Source: CAD feature listing. Evaluate the final solid. Frame: model axes, mm. Coordinates: 2 decimals unless noted, no trailing zeros. Loops run counter-clockwise (first coordinate to the right, second up) from the corner with the lowest first, then second, coordinate; pieces in that order, holes last. Notation, with made-up numbers: (-13.5, 16.25) -> (40.5, 16.25) arc R31 ccw to (40.5, 51.25) -> close; hole circle Ø11 at (-24, 13.5). An arc over 180 degrees is marked (long way). Answer as CSV lines item,"result".
from build123d import *

# Parameters (mm, degrees)
F1_DEPTH = 12
F3_DEPTH = 25
F5_D     = 5


with BuildPart() as f1:
    # F0 (on Front) → F1 (new body)
    with BuildSketch(Plane.XZ):
        with BuildLine():
            ThreePointArc((-6.1837801054, 11.6114190374), (-6.2418651063, 12.0437074429), (-6.411999761, 12.4453308138))
            ThreePointArc((-6.411999761, 12.4453308138), (-7.8214415512, 11.6114190374), (-9.1238598826, 10.6186242444))
            ThreePointArc((-9.1238598826, 10.6186242444), (-7.2975070499, 10.0598302873), (-6.1837801054, 11.6114190374))
        make_face()
        with BuildLine():
            ThreePointArc((-9.1238598826, 10.6186242444), (-5.8423437781, -12.7226970088), (14, 0))
            ThreePointArc((14, 0), (7.2880725623, 11.9534094854), (-6.411999761, 12.4453308138))
            ThreePointArc((-6.411999761, 12.4453308138), (-6.2418651063, 12.0437074429), (-6.1837801054, 11.6114190374))
            ThreePointArc((-6.1837801054, 11.6114190374), (-7.2975070499, 10.0598302873), (-9.1238598826, 10.6186242444))
        make_face()
    extrude(amount=F1_DEPTH)

    # F2 (on face) → F3 (cut)
    with BuildSketch(Plane.XZ.offset(12)):
        with BuildLine():
            ThreePointArc((-10.4471785382, 9.3196813567), (-8.7916106337, 8.9938043215), (-7.8551114747, 10.3973962329))
            ThreePointArc((-7.8551114747, 10.3973962329), (-7.9419845398, 10.903914247), (-8.1926740651, 11.3525367942))
            ThreePointArc((-8.1926740651, 11.3525367942), (-9.3751880821, 10.3973962329), (-10.4471785382, 9.3196813567))
        make_face()
        with BuildLine():
            ThreePointArc((-10.4471785382, 9.3196813567), (-9.3751880821, 10.3973962329), (-8.1926740651, 11.3525367942))
            ThreePointArc((-8.1926740651, 11.3525367942), (-10.393116946, 11.5263132895), (-10.4471785382, 9.3196813567))
        make_face()
        with BuildLine():
            ThreePointArc((-1.4187954682, 13.9279222937), (-2.9204529279, 13.692003312), (-4.3876813336, 13.2946700792))
            ThreePointArc((-4.3876813336, 13.2946700792), (-2.720036717, 12.1851966772), (-1.4003763205, 13.692003312))
            ThreePointArc((-1.4003763205, 13.692003312), (-1.4049881033, 13.810321771), (-1.4187954682, 13.9279222937))
        make_face()
        with BuildLine():
            ThreePointArc((-1.4187954682, 13.9279222937), (-3.237546655, 15.1786385936), (-4.3876813336, 13.2946700792))
            ThreePointArc((-4.3876813336, 13.2946700792), (-2.9204529279, 13.692003312), (-1.4187954682, 13.9279222937))
        make_face()
        with BuildLine():
            ThreePointArc((-13.7073626903, 2.847491541), (-13.3178491608, 4.3168152299), (-12.7713322624, 5.7352482286))
            ThreePointArc((-12.7713322624, 5.7352482286), (-14.7638599444, 4.7855216477), (-13.7073626903, 2.847491541))
        make_face()
        with BuildLine():
            ThreePointArc((-11.7977725535, 4.3168152299), (-12.0645773537, 5.1770144334), (-12.7713322624, 5.7352482286))
            ThreePointArc((-12.7713322624, 5.7352482286), (-13.3178491608, 4.3168152299), (-13.7073626903, 2.847491541))
            ThreePointArc((-13.7073626903, 2.847491541), (-12.3908803135, 3.112090511), (-11.7977725535, 4.3168152299))
        make_face()
        with BuildLine():
            ThreePointArc((5.7352482286, 12.7713322624), (4.3168152299, 13.3178491608), (2.847491541, 13.7073626903))
            ThreePointArc((2.847491541, 13.7073626903), (3.8481088121, 11.8718383773), (5.7352482286, 12.7713322624))
        make_face()
        with BuildLine():
            ThreePointArc((5.8368918373, 13.3178491608), (4.5132182902, 14.825184137), (2.847491541, 13.7073626903))
            ThreePointArc((2.847491541, 13.7073626903), (4.3168152299, 13.3178491608), (5.7352482286, 12.7713322624))
            ThreePointArc((5.7352482286, 12.7713322624), (5.8112649134, 13.0399048573), (5.8368918373, 13.3178491608))
        make_face()
        with BuildLine():
            ThreePointArc((-12.1719267046, -2.9204529279), (-12.7040716425, -1.7651936891), (-13.9279222937, -1.4187954682))
            ThreePointArc((-13.9279222937, -1.4187954682), (-13.692003312, -2.9204529279), (-13.2946700792, -4.3876813336))
            ThreePointArc((-13.2946700792, -4.3876813336), (-12.4848144608, -3.8442104556), (-12.1719267046, -2.9204529279))
        make_face()
        with BuildLine():
            ThreePointArc((11.3525367942, 8.1926740651), (10.3973962329, 9.3751880821), (9.3196813567, 10.4471785382))
            ThreePointArc((9.3196813567, 10.4471785382), (9.2684791764, 8.3572592183), (11.3525367942, 8.1926740651))
        make_face()
        with BuildLine():
            ThreePointArc((11.9174728403, 9.3751880821), (10.9772340204, 10.7803290119), (9.3196813567, 10.4471785382))
            ThreePointArc((9.3196813567, 10.4471785382), (10.3973962329, 9.3751880821), (11.3525367942, 8.1926740651))
            ThreePointArc((11.3525367942, 8.1926740651), (11.7689864991, 8.719922461), (11.9174728403, 9.3751880821))
        make_face()
        with BuildLine():
            ThreePointArc((-8.8773196255, -9.3751880821), (-9.7421306118, -8.003597816), (-11.3525367942, -8.1926740651))
            ThreePointArc((-11.3525367942, -8.1926740651), (-10.3973962329, -9.3751880821), (-9.3196813567, -10.4471785382))
            ThreePointArc((-9.3196813567, -10.4471785382), (-8.9922553032, -9.9550258696), (-8.8773196255, -9.3751880821))
        make_face()
        with BuildLine():
            ThreePointArc((13.9279222937, 1.4187954682), (13.692003312, 2.9204529279), (13.2946700792, 4.3876813336))
            ThreePointArc((13.2946700792, 4.3876813336), (12.2053680304, 2.6033592009), (13.9279222937, 1.4187954682))
        make_face()
        with BuildLine():
            ThreePointArc((15.2120799194, 2.9204529279), (14.6157608397, 4.1276417791), (13.2946700792, 4.3876813336))
            ThreePointArc((13.2946700792, 4.3876813336), (13.692003312, 2.9204529279), (13.9279222937, 1.4187954682))
            ThreePointArc((13.9279222937, 1.4187954682), (14.8472625508, 1.9325212585), (15.2120799194, 2.9204529279))
        make_face()
        with BuildLine():
            ThreePointArc((-2.7967386225, -13.3178491608), (-4.0388709263, -11.8233994774), (-5.7352482286, -12.7713322624))
            ThreePointArc((-5.7352482286, -12.7713322624), (-4.3168152299, -13.3178491608), (-2.847491541, -13.7073626903))
            ThreePointArc((-2.847491541, -13.7073626903), (-2.8094802537, -13.5142522211), (-2.7967386225, -13.3178491608))
        make_face()
        with BuildLine():
            ThreePointArc((4.3876813336, -13.2946700792), (2.9204529279, -13.692003312), (1.4187954682, -13.9279222937))
            ThreePointArc((1.4187954682, -13.9279222937), (3.0387713869, -15.2074681366), (4.4405295353, -13.692003312))
            ThreePointArc((4.4405295353, -13.692003312), (4.4272595627, -13.4915871011), (4.3876813336, -13.2946700792))
        make_face()
        with BuildLine():
            ThreePointArc((4.3876813336, -13.2946700792), (2.6033592009, -12.2053680304), (1.4187954682, -13.9279222937))
            ThreePointArc((1.4187954682, -13.9279222937), (2.9204529279, -13.692003312), (4.3876813336, -13.2946700792))
        make_face()
        with BuildLine():
            ThreePointArc((12.7713322624, -5.7352482286), (13.3178491608, -4.3168152299), (13.7073626903, -2.847491541))
            ThreePointArc((13.7073626903, -2.847491541), (11.8718383773, -3.8481088121), (12.7713322624, -5.7352482286))
        make_face()
        with BuildLine():
            ThreePointArc((14.8379257682, -4.3168152299), (14.5225738798, -3.3898463825), (13.7073626903, -2.847491541))
            ThreePointArc((13.7073626903, -2.847491541), (13.3178491608, -4.3168152299), (12.7713322624, -5.7352482286))
            ThreePointArc((12.7713322624, -5.7352482286), (14.1780483644, -5.570087037), (14.8379257682, -4.3168152299))
        make_face()
        with BuildLine():
            ThreePointArc((10.4471785382, -9.3196813567), (8.3572592183, -9.2684791764), (8.1926740651, -11.3525367942))
            ThreePointArc((8.1926740651, -11.3525367942), (9.3751880821, -10.3973962329), (10.4471785382, -9.3196813567))
        make_face()
    extrude(amount=-F3_DEPTH, mode=Mode.SUBTRACT)

    # F5 (through all)
    with Locations(Plane(origin=(0, 0, 0), x_dir=(-1, 0, 0), z_dir=(0, 1, 0))):
        with Locations((0, 0)):
            Hole(F5_D / 2)


solid = f1.part
(1) Material intervals for L1, parallel to Z at x = 0, y = -9; L2, parallel to X at y = -8.5, z = 0.75; L3, parallel to Z at x = -7.25, y = -8.25, sorted ascending. Write a range as [from, to].
Computed values:
L1,"[-14, -2.5], [2.5, 14]"
L2,"[-13.98, -2.38], [2.38, 13.98]"
L3,"[-11.98, 11.98]"
(2) Cut plane D-D (x = 5). Return the cut outline in (y, z), then the cut area to 3 significant figures.
Computed values:
outline,"(-12, -13.08) -> (0, -13.08) -> (0, 11.96) -> (-12, 11.96) -> close"
area,"300 mm^2"
(3) Cut plane B-B (y = -3.5). Return the cut outline in (x, z).
Computed values:
outline,"(-13.93, -1.42) arc R1.52 cw to (-13.29, -4.39) arc R14 ccw to (-11.35, -8.19) arc R1.52 cw to (-9.32, -10.45) arc R14 ccw to (-5.74, -12.77) arc R1.52 cw to (-2.85, -13.71) arc R14 ccw to (1.42, -13.93) arc R1.52 cw to (4.39, -13.29) arc R14 ccw to (8.19, -11.35) arc R1.52 cw to (10.45, -9.32) arc R14 ccw to (12.77, -5.74) arc R1.52 cw to (13.71, -2.85) arc R14 ccw to (13.93, 1.42) arc R1.52 cw to (13.29, 4.39) arc R14 ccw to (11.35, 8.19) arc R1.52 cw to (9.32, 10.45) arc R14 ccw to (5.74, 12.77) arc R1.52 cw to (2.85, 13.71) arc R14 ccw to (-1.42, 13.93) arc R1.52 cw to (-4.39, 13.29) arc R14 ccw to (-8.19, 11.35) arc R1.52 cw to (-10.45, 9.32) arc R14 ccw to (-12.77, 5.74) arc R1.52 cw to (-13.71, 2.85) arc R14 ccw to start; hole circle Ø5 at (0, 0)"
(4) Draft query along X for faces 1 (the cylindrical face through (9.25, -6.08, 8.38)), 2 (the cylindrical face through (-7.64, -5.92, -11.73)), 3 (the cylindrical face through (7.64, -5.92, 11.73)). Return one class per face: released by +X, released by -X, zero draft, split by the parting line, or undercut.
Computed values:
face 1,"undercut"
face 2,"released by -X"
face 3,"released by +X"
(5) Cut plane C-C (z = -2). Return the cut outline in (x, y).
Computed values:
outline,"(-12.48, -12) -> (-1.5, -12) -> (-1.5, 0) -> (-12.48, 0) -> close; (1.5, -12) -> (13.86, -12) -> (13.86, 0) -> (1.5, 0) -> close"
(6) Cut plane A-A (x = 0). Return the cut outline in (y, z), then the cut area to 3 significant figures.
Computed values:
outline,"(-12, -14) -> (0, -14) -> (0, -2.5) -> (-12, -2.5) -> close; (-12, 2.5) -> (0, 2.5) -> (0, 14) -> (-12, 14) -> close"
area,"276 mm^2"
(7) Pin query (flat end, axial travel): pin 1 Ø1 at (x, y) = (6, -10.5) entering from +Z. Return the tip coordinate at first contact, or that it passes through.
Computed values:
pin 1,"z = 12.77"
